```python
from build123d import *

# Parameters (mm, degrees)
FILLET_1_R          = 0.3
CUT_EXTRUDE_1_DEPTH = 2.4
CHAMFER_1_SIZE      = 0.2


with BuildPart() as part:
    # 草图1 → 旋转1 (revolve)
    with BuildSketch(Plane.XY):
        Polygon((0, 3.5), (-3.5, 3.5), (-3.5, 0), (-2, 0), (-2, -5), (-1.5, -5), (-1.5, -10.5), (0, -10.5), align=None)
    revolve(axis=Axis((0, 3.5, 0), (0, -1, 0)))

    # 圆角1
    fillet_1_edges = [part.edges().sort_by_distance(p)[0] for p in [
        (3.5, 0, 0),
        (3.5, 3.5, 0),
    ]]
    fillet(fillet_1_edges, radius=FILLET_1_R)

    # 草图2 → 切除-拉伸1 (cut)
    with BuildSketch(Plane(origin=(0, 3.5, 0), x_dir=(1, 0, 0), z_dir=(0, 1, 0))):
        Polygon((1.5, -0.866025404), (1.5, 0.866025404), (0, 1.732050808), (-1.5, 0.866025404), (-1.5, -0.866025404), (0, -1.732050808), align=None)
    extrude(amount=-CUT_EXTRUDE_1_DEPTH, mode=Mode.SUBTRACT)

    # 倒角1
    chamfer_1_edges = [part.edges().sort_by_distance(p)[0] for p in [
        (2, -5, 0),
    ]]
    chamfer(chamfer_1_edges, length=CHAMFER_1_SIZE)


solid = part.part
```
Can you work these out from the model? Positions are in its coordinate system, mm. A direction names the side the tool comes from. Coordinates: 2 decimals unless noted, no trailing zeros. Loops run counter-clockwise (first coordinate to the right, second up) from the corner with the lowest first, then second, coordinate; pieces in that order, holes last.
1) For pin 1 (1 mm diameter, centred on y = 1, z = 1, fed in from +X); pin 2 (1 mm diameter, centred on x = -1.5, y = 1.5, fed in from +Z); pin 3 (1 mm diameter, centred on y = 1, z = 2.5, fed in from +X), each with a flat end and sliding along its axis, tell me the tip position at first contact or that it passes through.
2) Imagine slicing it at A-A on z = 0. List the corners of the cut face in (x, y) for me, plus the area to 3 significant figures.
3) I need wall thicknesses on probe 1 along Y at (x, z) = (-0.75, -1.5); probe 2 along Y at (x, z) = (-2, -1.5); probe 3 along Z at (x, y) = (-1, -2.75). Which ranges of each line are inside material? Lowest first, please.
4) Imagine slicing it at B-B on y = -8.25. List the corners of the cut face in (x, z) for me.
5) Which directions (+Z, -Z, +X, -X, +Y, -Y) give clear straight access to the entire face, cutting with the end or side of a thin tool? Please do faces 1 (the flat face through (-0.74, 2.317, -1.305)), 2 (the cylindrical face through (1.5, -7.79, -0.07)), 3 (the flat face through (0, -10.5, 0)).
6) Thinking about a two-plate mould opening in Z: for faces 4 (the cylindrical face through (0, -2, 2)), 5 (the flat face through (-0.76, 2.317, 1.293)), 6 (the flat face through (-2, 0, 1)), which applies, pulls with the +Z half, pulls with the -Z half, needs draft (parallel to the pull), parting line crosses it, or undercut?
Completed:
1. pin 1: stops at x = 3.46
1. pin 2: stops at z = 3.35
1. pin 3: stops at x = 2.87
2. outline: (-3.5, 0.3) arc R0.3 ccw to (-3.2, 0) - (-2, 0) - (-2, -4.8) - (-1.8, -5) - (-1.5, -5) - (-1.5, -10.5) - (1.5, -10.5) - (1.5, -5) - (1.8, -5) - (2, -4.8) - (2, 0) - (3.2, 0) arc R0.3 ccw to (3.5, 0.3) - (3.5, 3.2) arc R0.3 ccw to (3.2, 3.5) - (1.5, 3.5) - (1.5, 1.1) - (-1.5, 1.1) - (-1.5, 3.5) - (-3.2, 3.5) arc R0.3 ccw to (-3.5, 3.2) - close
2. area: 53.7 mm2
3. probe 1: y = -5 to 3.5
3. probe 2: y = 0 to 3.5
3. probe 3: z = -1.73 to 1.73
4. outline: circle Ø3 at (0, 0)
5. face 1: +Y
5. face 2: -Y
5. face 3: +Z, -Z, +X, -X, -Y
6. face 4: parting line crosses it
6. face 5: undercut
6. face 6: needs draft
